Check sheet for the modelled part. Datum: model origin and axes. Units: mm. A direction names the side the tool comes from. Round coordinates to 2 decimals unless told otherwise and drop trailing zeros. Write each loop counter-clockwise with the first axis right and the second up, starting at its lowest first coordinate (ties: lowest second). Pieces come first, ordered by that corner, then holes. Notation, with made-up numbers: (-6, 18.5) -> (6, 18.5) arc R21 cw to (6, 36.5) -> close; hole circle Ø2 at (29.5, 56). An arc over 180 degrees is marked (long way). Write item = value, one per line.
from build123d import *

# Parameters (mm, degrees)
REFRENTADO_PARA_TORNILLO_CON_CABEZA_HUEC_D           = 6.6
REFRENTADO_PARA_TORNILLO_CON_CABEZA_HUEC_CBORE_D     = 11
REFRENTADO_PARA_TORNILLO_CON_CABEZA_HUEC_CBORE_DEPTH = 36.4


with BuildPart() as part:
    # Croquis1 → Revolución1 (revolve)
    with BuildSketch(Plane.XY, mode=Mode.PRIVATE) as revoluci_n1_sk:
        Polygon((0, 50), (0, 0), (25.4, 0), (25.4, 30), (12.7, 30), (12.7, 50), align=None)
    revolve(revoluci_n1_sk.sketch.rotate(Axis((0, 50, 0), (0, -1, 0)), 90), axis=Axis((0, 50, 0), (0, -1, 0)))

    # Refrentado para tornillo con cabeza hueca de M61 (through all)
    with Locations(Plane(origin=(0, 50, 0), x_dir=(1, 0, 0), z_dir=(0, 1, 0))):
        with Locations((0, 0)):
            CounterBoreHole(REFRENTADO_PARA_TORNILLO_CON_CABEZA_HUEC_D / 2, REFRENTADO_PARA_TORNILLO_CON_CABEZA_HUEC_CBORE_D / 2, REFRENTADO_PARA_TORNILLO_CON_CABEZA_HUEC_CBORE_DEPTH)


solid = part.part
(1) Release check for a two-part mould opening along X. For faces 3 (the flat face through (3, 50, 5)), 4 (the cylindrical face through (15.456, 15.21, -20.157)), 5 (the cylindrical face through (-1.19, 32.05, 5.37)) record: pulls with the +X half, pulls with the -X half, needs draft (parallel to the pull), parting line crosses it, or undercut.
Worked answers:
face_3 = needs draft
face_4 = parting line crosses it
face_5 = undercut
(2) Sectioned sample at D-D on x = 7. Enter the section's corners in (y, z), then the cut area to 3 significant figures.
Worked answers:
outline = (0, -24.42) -> (30, -24.42) -> (30, -10.6) -> (50, -10.6) -> (50, 10.6) -> (30, 10.6) -> (30, 24.42) -> (0, 24.42) -> close
area = 1,890 mm²
(3) Go/stop test with flat-tipped pins: P1, Ø8, axis at y = 12.5, z = 12, coming from the +X side; P2, Ø10, axis at x = 2, z = 19, coming from the +Y side; P3, Ø17.5, axis at x = 0, z = 0, coming from the +Y side; P4, Ø5, axis at y = 27, z = -2, coming from the +X side. Record where each tip stops, or that it passes through.
Worked answers:
P1 = 24.11
P2 = 30
P3 = 50
P4 = 25.4
(4) Sectioned sample at C-C on y = 25. Enter the section's corners in (x, z).
Worked answers:
outline = circle Ø50.8 at (0, 0); hole circle Ø11 at (0, 0)
(5) Sectioned sample at A-A on z = 0. Enter the section's corners in (x, y).
Worked answers:
outline = (-25.4, 0) -> (-3.3, 0) -> (-3.3, 13.6) -> (-5.5, 13.6) -> (-5.5, 50) -> (-12.7, 50) -> (-12.7, 30) -> (-25.4, 30) -> close; (3.3, 0) -> (25.4, 0) -> (25.4, 30) -> (12.7, 30) -> (12.7, 50) -> (5.5, 50) -> (5.5, 13.6) -> (3.3, 13.6) -> close
(6) Material ranges on L1, parallel to Y at x = 21.5, z = -10; L2, parallel to Z at x = 3, y = 22; L3, parallel to Z at x = -4.5, y = 45, recorded low to high. Write a range as [from, to].
Worked answers:
L1 = [0, 30]
L2 = [-25.22, -4.61], [4.61, 25.22]
L3 = [-11.88, -3.16], [3.16, 11.88]
(7) Access from +Z, -Z, +X, -X, +Y, -Y to the whole of each face (thin tool, end or side, straight path). Record for faces 1 (the flat face through (0, 0, -5)), 2 (the cylindrical face through (7.7, 40.1, -10.1)).
Worked answers:
face_1 = +Z, -Z, +X, -X, -Y
face_2 = +Y
(8) Sectioned sample at B-B on x = 0. Enter the section's corners in (y, z).
Worked answers:
outline = (0, -25.4) -> (30, -25.4) -> (30, -12.7) -> (50, -12.7) -> (50, -5.5) -> (13.6, -5.5) -> (13.6, -3.3) -> (0, -3.3) -> close; (0, 3.3) -> (13.6, 3.3) -> (13.6, 5.5) -> (50, 5.5) -> (50, 12.7) -> (30, 12.7) -> (30, 25.4) -> (0, 25.4) -> close
